Drawing for the job (mm, zero at the part's lowest x, y, z). Give positions to 0.01 mm unless a question says otherwise; leave off trailing zeros. Order: outer loops, then holes, each group sorted by start corner. A loop starts at its lowest first (then second) coordinate and runs counter-clockwise, first axis right, second up. Notation, with made-up numbers: (59.5, -29.5) - (92.5, -29.5) arc R16 ccw to (92.5, -1.5) - close; hole circle Ø6 at (47.25, 77). An arc over 180 degrees is marked (long way). Use a Markdown table: item, result. Add a question column.
(1) Wall check: line 1 (X direction, y = 0.95, z = 5); line 2 (Z direction, x = 4, y = 3.7) (1 decimal); line 3 (Y direction, x = 3.2, z = 27.75). Give the ranges that are in metal, low to high.
(2) Slice it at A-A (x = 3.5). Write the cut outline in (y, z).
(3) Flat gauge pins, fed straight in: pin 1 (3 mm diameter, centred on y = 3, z = 27.75, fed in from -X); pin 2 (0.6 mm diameter, centred on y = 3, z = 3.5, fed in from -X); pin 3 (0.6 mm diameter, centred on y = 2.5, z = 52, fed in from -X); pin 4 (1 mm diameter, centred on x = 15.5, y = 4, fed in from -Z). Where does each tip first touch, or does it go through?
(4) Slice it at B-B (z = 21.5). Write the cut outline in (x, y).
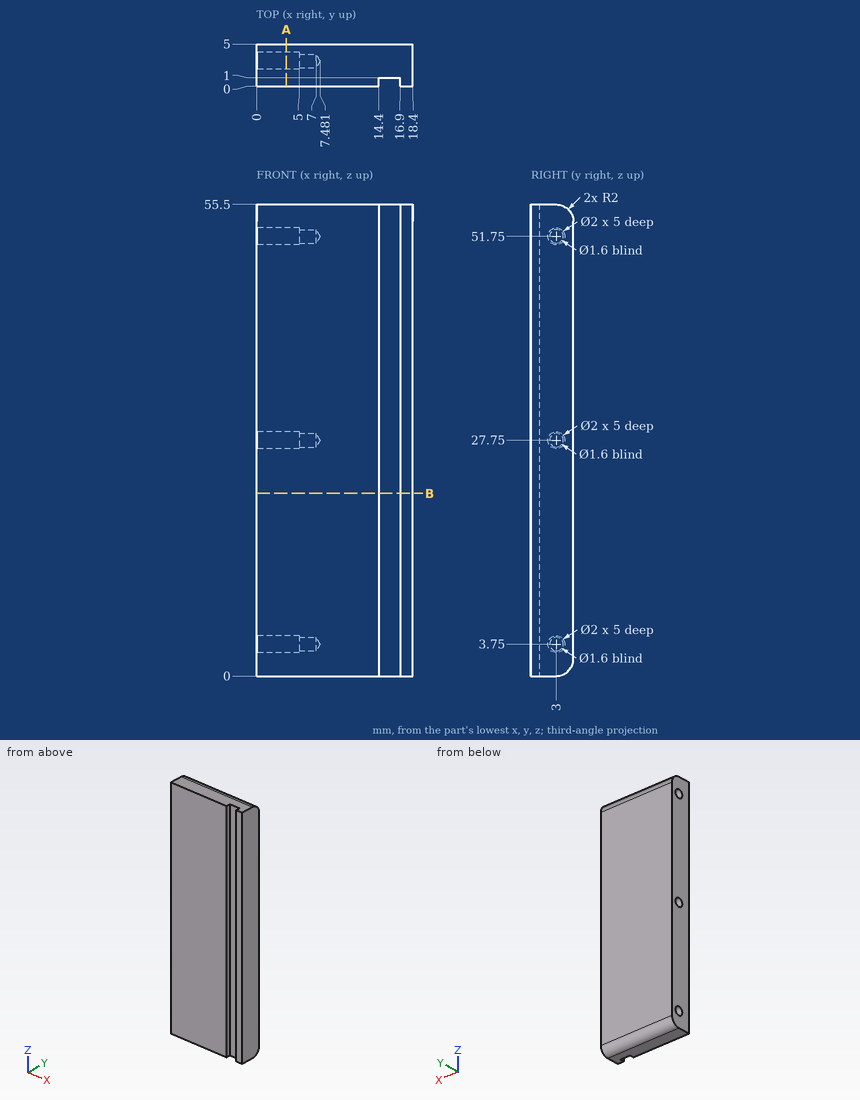
Solution:
| question | item | result |
|---|---|---|
| 1 | line 1 | 0 to 14.4, 16.9 to 18.4 |
| 1 | line 2 | 0.1 to 3, 4.5 to 27, 28.5 to 51, 52.5 to 55.4 |
| 1 | line 3 | 0 to 2, 4 to 5 |
| 2 | outline | (0, 0) - (3, 0) arc R2 ccw to (5, 2) - (5, 53.5) arc R2 ccw to (3, 55.5) - (0, 55.5) - close; hole circle Ø2 at (3, 3.75); hole circle Ø2 at (3, 27.75); hole circle Ø2 at (3, 51.75) |
| 3 | pin 1 | x = 0 |
| 3 | pin 2 | x = 7.15 |
| 3 | pin 3 | x = 5 |
| 3 | pin 4 | z = 0.06 |
| 4 | outline | (0, 0) - (14.4, 0) - (14.4, 1) - (16.9, 1) - (16.9, 0) - (18.4, 0) - (18.4, 5) - (0, 5) - close |
